```python
from build123d import *

# Parameters (mm, degrees)
CROQUIS2_W                    = 23.9
CROQUIS2_H                    = 12.5
SALIENTE_EXTRUIR1_DEPTH       = 0.9
CROQUIS4_W                    = 17.8
CROQUIS4_H                    = 4
SALIENTE_EXTRUIR2_DEPTH       = 1
CROQUIS5_W                    = 8
CROQUIS5_H                    = 4
SALIENTE_EXTRUIR3_DEPTH       = 4.2
CROQUIS6_W                    = 5.2
CROQUIS6_H                    = 11
SALIENTE_EXTRUIR4_DEPTH       = 2.8
DI_METRO_DE_TALADRO_2_0_2_1_D = 2


with BuildPart() as part:
    # Croquis2 → Saliente-Extruir1 (new body)
    with BuildSketch(Plane.XY):
        with Locations((0.45, 6.25)):
            Rectangle(CROQUIS2_W, CROQUIS2_H)
    saliente_extruir1 = extrude(amount=SALIENTE_EXTRUIR1_DEPTH)

    # Croquis4 → Saliente-Extruir2 (add)
    with BuildSketch(Plane.XY.offset(0.9)):
        with Locations((2.5, 2)):
            Rectangle(CROQUIS4_W, CROQUIS4_H)
    saliente_extruir2 = extrude(amount=SALIENTE_EXTRUIR2_DEPTH)

    # Croquis5 → Saliente-Extruir3 (add)
    with BuildSketch(Plane.XY.offset(1.9)):
        with Locations((-2.4, 2)):
            Rectangle(CROQUIS5_W, CROQUIS5_H)
    saliente_extruir3 = extrude(amount=SALIENTE_EXTRUIR3_DEPTH)

    # Croquis6 → Saliente-Extruir4 (add)
    with BuildSketch(Plane(origin=(0, 0, 0), x_dir=(-1, 0, 0), z_dir=(0, 0, -1))):
        with Locations((8.9, 5.5)):
            Rectangle(CROQUIS6_W, CROQUIS6_H)
    saliente_extruir4 = extrude(amount=SALIENTE_EXTRUIR4_DEPTH)

    # Diámetro de taladro Ø2.0 (2)1 (through all)
    with Locations(Plane(origin=(-2.15, 10.5, 0.9), x_dir=(1, 0, 0), z_dir=(0, 0, 1))):
        with Locations((0, 0), (12.5, 0)):
            di_metro_de_taladro_2_0_2_1 = Hole(DI_METRO_DE_TALADRO_2_0_2_1_D / 2)

    # Simetría1: Saliente-Extruir1, Saliente-Extruir2, Saliente-Extruir3, Saliente-Extruir4 across plane
    add(saliente_extruir1.mirror(Plane.ZX))
    add(saliente_extruir2.mirror(Plane.ZX))
    add(saliente_extruir3.mirror(Plane.ZX))
    add(saliente_extruir4.mirror(Plane.ZX))

    # Simetría2: Diámetro de taladro Ø2.0 (2)1 across plane
    add(di_metro_de_taladro_2_0_2_1.mirror(Plane.ZX), mode=Mode.SUBTRACT)


solid = part.part
```
Work out the finished part from the listing and answer in its coordinate system (mm). A direction names the side the tool comes from. Give positions to 0.01 mm unless a question says otherwise; leave off trailing zeros. Order: outer loops, then holes, each group sorted by start corner. A loop starts at its lowest first (then second) coordinate and runs counter-clockwise, first axis right, second up.
1. Each of these flat-tipped pins is pushed along its axis until it touches: P1, Ø4, axis at x = 8, y = 9, coming from the +Z side; P2, Ø4, axis at y = 2, z = 4.5, coming from the -X side; P3, Ø1.3, axis at y = -0.5, z = 4.5, coming from the +X side. Where does it stop, or does it pass through?
Result sheet:
P1: stops at z = 0.9
P2: stops at x = -6.4
P3: stops at x = 1.6
2. For faces 1 (the flat face through (6, 0, 1.9)), 2 (the flat face through (-9, -11, -1)), 3 (the flat face through (-6.4, 0, 3)), determine the directions among +Z, -Z, +X, -X, +Y, -Y from which every point of the face is accessible in a straight line to the end or side of a thin tool.
Result sheet:
face 1: +Z, +X, +Y, -Y
face 2: -Z, +X, -X, -Y
face 3: +Z, -X, +Y, -Y
3. Straight lines are drawn through the part: L1, parallel to Y at x = 10.35, z = 0.4; L2, parallel to X at y = -5.75, z = -2; L3, parallel to Z at x = 3.5, y = -3.75. For each, find the intervals that lie inside material, in ascending order.
Result sheet:
L1: y = -12.5 to -11.5, -9.5 to 9.5, 11.5 to 12.5
L2: x = -11.5 to -6.3
L3: z = 0 to 1.9
4. Section A-A, the plane x = 10.35 is taken. Determine the outline of the cut face in (y, z), and give its area (3 significant figures).
Result sheet:
outline: (-12.5, 0) - (-11.5, 0) - (-11.5, 0.9) - (-12.5, 0.9) - close; (-9.5, 0) - (9.5, 0) - (9.5, 0.9) - (4, 0.9) - (4, 1.9) - (-4, 1.9) - (-4, 0.9) - (-9.5, 0.9) - close; (11.5, 0) - (12.5, 0) - (12.5, 0.9) - (11.5, 0.9) - close
area: 26.9 mm2
5. Section D-D, the plane y = -5 is taken. Determine the outline of the cut face in (x, z), and give its area (3 significant figures).
Result sheet:
outline: (-11.5, -2.8) - (-6.3, -2.8) - (-6.3, 0) - (12.4, 0) - (12.4, 0.9) - (-11.5, 0.9) - close
area: 36.1 mm2
6. Section C-C, the plane x = 2 is taken. Determine the outline of the cut face in (y, z), and give its area (3 significant figures).
Result sheet:
outline: (-12.5, 0) - (12.5, 0) - (12.5, 0.9) - (4, 0.9) - (4, 1.9) - (-4, 1.9) - (-4, 0.9) - (-12.5, 0.9) - close
area: 30.5 mm2
7. Section B-B, the plane y = -10 is taken. Determine the outline of the cut face in (x, z).
Result sheet:
outline: (-11.5, -2.8) - (-6.3, -2.8) - (-6.3, 0) - (-3.02, 0) - (-3.02, 0.9) - (-11.5, 0.9) - close; (-1.28, 0) - (9.48, 0) - (9.48, 0.9) - (-1.28, 0.9) - close; (11.22, 0) - (12.4, 0) - (12.4, 0.9) - (11.22, 0.9) - close
8. The mould has two halves that part along Y. Classify faces 4 (the flat face through (-6.3, 0, -1)), 5 (the flat face through (-2, 4, 3)), 6 (the flat face through (-2, -4, 3)), 7 (the cylindrical face through (-2.69, 11.34, 0.44)): released by +Y, released by -Y, zero draft, split by the parting line, or undercut.
Result sheet:
face 4: zero draft
face 5: released by +Y
face 6: released by -Y
face 7: undercut
